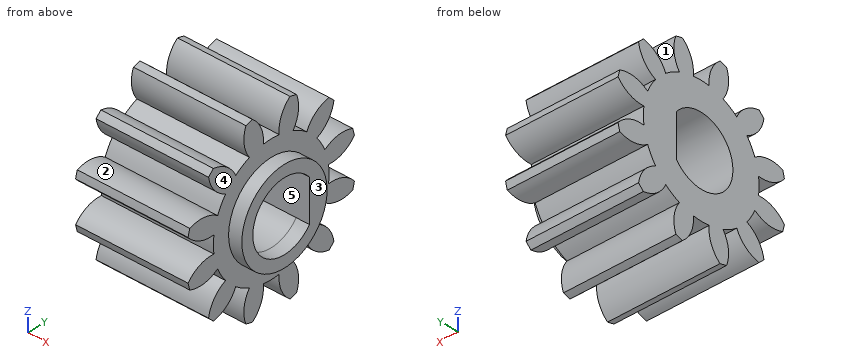
from build123d import *

# Parameters (mm, degrees)
BASPROSKE_W         = 8.5
BASPROSKE_H         = 7
TOOTHCUT_DEPTH      = 14.047988351
TEETHCUTS_COUNT     = 12
TEETHCUTS_ANGLE     = 330
BORSKE_R            = 2.6
BORE_DEPTH          = 50.0000508
BOSS_EXTRUDE1_DEPTH = 8.5
SKETCH2_R           = 3.5
BOSS_EXTRUDE2_DEPTH = 1


with BuildPart() as part:
    # BasProSke → Base-Revolve (revolve)
    with BuildSketch(Plane(origin=(0, 0, 0), x_dir=(1, 0, 0), z_dir=(0, 1, 0)), mode=Mode.PRIVATE) as base_revolve_sk:
        with Locations((4.25, 3.5)):
            Rectangle(BASPROSKE_W, BASPROSKE_H)
    revolve(base_revolve_sk.sketch.rotate(Axis((-10, 0, 0), (1, 0, 0)), 180), axis=Axis((-10, 0, 0), (1, 0, 0)))

    # TooCutSke → ToothCut (cut, through all)
    with BuildSketch(Plane(origin=(0, 0, 0), x_dir=(0, 0, -1), z_dir=(1, 0, 0))):
        with BuildLine():
            ThreePointArc((0.649675465, 4.704351474), (0, 4.749), (-0.649675465, 4.704351474))
            ThreePointArc((-0.649675465, 4.704351474), (-0.830100462, 5.895273832), (-1.56637772, 6.84855503))
            ThreePointArc((-1.56637772, 6.84855503), (0, 7.0254), (1.56637772, 6.84855503))
            ThreePointArc((1.56637772, 6.84855503), (0.830100462, 5.895273832), (0.649675465, 4.704351474))
        make_face()
    toothcut = extrude(amount=TOOTHCUT_DEPTH, mode=Mode.SUBTRACT)

    # TeethCuts: ToothCut ×12 about axis
    teethcuts_axis = Axis((-10, 0, 0), (1, 0, 0))
    for i in range(1, TEETHCUTS_COUNT):
        add(toothcut.rotate(teethcuts_axis, i * TEETHCUTS_ANGLE / (TEETHCUTS_COUNT - 1)), mode=Mode.SUBTRACT)

    # BorSke → Bore (cut, symmetric)
    with BuildSketch(Plane(origin=(0, 0, 0), x_dir=(0, 0, -1), z_dir=(1, 0, 0))):
        with Locations(Location((0, 0, 0), (0, 0, 180))):
            Circle(BORSKE_R)
    extrude(amount=BORE_DEPTH, both=True, mode=Mode.SUBTRACT)

    # Sketch1 → Boss-Extrude1 (add)
    with BuildSketch(Plane(origin=(8.5, 0, 0), x_dir=(0, 0, -1), z_dir=(1, 0, 0))):
        with BuildLine():
            Line((-1.599218559, 2.05), (1.599218559, 2.05))
            ThreePointArc((1.599218559, 2.05), (0, 2.6), (-1.599218559, 2.05))
        make_face()
    extrude(amount=-BOSS_EXTRUDE1_DEPTH)

    # Sketch2 → Boss-Extrude2 (add)
    with BuildSketch(Plane(origin=(8.5, 0, 0), x_dir=(0, 0, -1), z_dir=(1, 0, 0))):
        with Locations(Location((0, 0, 0), (0, 0, 180))):
            Circle(SKETCH2_R)
        with BuildLine():
            Line((-1.599218559, 2.05), (1.599218559, 2.05))
            ThreePointArc((1.599218559, 2.05), (0, -2.6), (-1.599218559, 2.05))
        make_face(mode=Mode.SUBTRACT)
    extrude(amount=BOSS_EXTRUDE2_DEPTH)


solid = part.part
The model under review builds one solid part; all positions refer to its coordinate system, in mm. Face numbers are marked on the shaded views. A direction names the side the tool comes from. Round coordinates to 2 decimals unless told otherwise and drop trailing zeros. Loops run counter-clockwise (first coordinate to the right, second up) from the corner with the lowest first, then second, coordinate; pieces in that order, holes last. Notation, with made-up numbers: M -20.5,-35 L -14.5,-35 A20 cw -14.5,-3 Z; hole C 67,68.5 d3. An arc over 180 degrees is marked long. Answer as a JSON object with one key per item and string values.
Item 1: We need section B-B, the plane z = 0. State the section outline as (x, y) points, and give its area (3 significant figures).
Check sheet entries:
{"outline": "M 0,-4.75 L 8.5,-4.75 L 8.5,-3.5 L 9.5,-3.5 L 9.5,-2.6 L 0,-2.6 Z; M 0,2.05 L 9.5,2.05 L 9.5,3.5 L 8.5,3.5 L 8.5,4.75 L 0,4.75 Z", "area": "43.6 mm2"}
Item 2: We need section C-C, the plane y = 2.5. State the section outline as (x, z) points.
Check sheet entries:
{"outline": "M 0,-4.04 L 8.5,-4.04 L 8.5,-2.45 L 9.5,-2.45 L 9.5,2.45 L 8.5,2.45 L 8.5,4.04 L 0,4.04 Z"}
Item 3: Clearance check with flat-ended pins moving along their axes: P1, Ø5, axis at y = 5, z = 4, coming from the +X side; P2, Ø2, axis at x = 7.5, y = 3.5, coming from the +Z side; P3, Ø4, axis at y = 0, z = 0, coming from the +X side; P4, Ø3, axis at x = 1, z = -3.5, coming from the +Y side. State where each tip first meets the part, or that it passes through.
Check sheet entries:
{"P1": "x = 8.5", "P2": "z = 5.09", "P3": "through", "P4": "y = 6.71"}
Item 4: For line 1 along Y through (x, z) = (5.75, 0); line 2 along Z through (x, y) = (4.5, 0); line 3 along Z through (x, y) = (7, 4.25), list the stretches that pass through material, from the lowest coordinate up.
Check sheet entries:
{"line 1": "-4.75 to -2.6, 2.05 to 4.75", "line 2": "-4.75 to -2.6, 2.6 to 4.75", "line 3": "-5.01 to -3.22, -2.12 to 2.12, 3.22 to 5.01"}
Item 5: The part is to be moulded in two halves that separate along Y. For the marked faces 1, 2 and 3, say which applies: +Y half, -Y half, draft (parallel to the pull), parting line (faces both ways), or undercut.
Check sheet entries:
{"face 1": "undercut", "face 2": "undercut", "face 3": "draft"}
Item 6: We need section A-A, the plane y = 0. State the section outline as (x, z) points.
Check sheet entries:
{"outline": "M 0,-4.75 L 8.5,-4.75 L 8.5,-3.5 L 9.5,-3.5 L 9.5,-2.6 L 0,-2.6 Z; M 0,2.6 L 9.5,2.6 L 9.5,3.5 L 8.5,3.5 L 8.5,4.75 L 0,4.75 Z"}
Item 7: Tool access review of the marked faces 4 and 5: name each direction out of +Z, -Z, +X, -X, +Y, -Y from which nothing blocks a thin tool from reaching the whole face with its end or side.
Check sheet entries:
{"face 4": "+X", "face 5": "+X, -X"}
